The listing builds one solid part. Answer for the finished solid, in the listing's coordinates (mm). Face numbers are marked on the shaded views. A direction names the side the tool comes from. Coordinates: 2 decimals unless noted, no trailing zeros. Write each loop counter-clockwise with the first axis right and the second up, starting at its lowest first coordinate (ties: lowest second). Pieces come first, ordered by that corner, then holes.
(1) For a pull along Z with two mould halves and no side action, classify the marked faces 1, 2 and 3 as +Z half, -Z half, draft (parallel to the pull), parting line (faces both ways), or undercut.
(2) Which of the six approach directions +Z, -Z, +X, -X, +Y, -Y give full straight-line access (tool end or side, diameter ignored) to the marked faces 4 and 5?
(3) The part is cut by section A-A on x = -0.5. Determine the outline of the cut face in (y, z), plus the area to 3 significant figures.
(4) Straight lines are drawn through the part: line 1 (Z direction, x = -1, y = 0); line 2 (X direction, y = -5, z = 10.75). For each, find the intervals that lie inside material, in ascending order.
(5) Given P1, Ø9.5, axis at y = 2.5, z = 0.5, coming from the +X side; P2, Ø6, axis at x = 9, z = 0, coming from the -Y side; P3, Ø12, axis at x = 6, z = -10.5, coming from the -Y side; P4, Ø6, axis at x = 3, z = 9, coming from the -Y side, each flat-ended and moving along its own axis, determine where each tip first touches the part or whether it passes through.
from build123d import *

# Parameters (mm, degrees)
SKETCH_2_R      = 6.3
EXTRUDE_1_DEPTH = 1


with BuildPart() as part:
    # Эскиз1 → Повернуть-Тонкостенный3 (revolve)
    with BuildSketch(Plane.XY):
        Polygon((-41.34237999, 7), (16.65762001, 7), (19.313431248, 2.4), (27.313431248, 2.120633844), (27.2890016, 1.421060265), (18.901221633, 1.713967996), (16.253474821, 6.3), (-41.34237999, 6.3), align=None)
    revolve(axis=Axis((-11.565290599, 0, 0), (1, 0, 0)))

    # Эскиз2 → Бобышка-Вытянуть1 (add)
    with BuildSketch(Plane.ZY.offset(41.34237999)):
        with BuildLine():
            add(Edge.make_bspline(
                [(-14.5, 0), (-14.474728727, -1.250629482), (-14.242328004, -3.018058456), (-13.480726208, -5.156192857), (-12.386888331, -6.242148201), (-11.142838362, -6.727444369), (-9.562420274, -7.125179123), (-7.483693891, -7.691921698), (-4.724391308, -8.363720089), (-2.266989559, -9.122366404), (-0.655182959, -9.33281469), (-0.082845288, -9.355711433), (-2e-08, -9.357888542)],
                knots=[0, 0, 0, 0, 0.178779937, 0.255445115, 0.319697761, 0.392573489, 0.443879083, 0.553726464, 0.701162756, 0.851190942, 0.921407161, 0.933286403, 0.933286403, 0.933286403, 0.933286403], degree=3))
            add(Edge.make_bspline(
                [(14.5, 0), (14.474728734, -1.250629483), (14.242328006, -3.018058455), (13.480726218, -5.156192862), (12.386888336, -6.242148209), (11.142838364, -6.727444374), (9.562420275, -7.125179117), (7.483693885, -7.691921727), (4.724391348, -8.363719948), (2.266989446, -9.122366813), (0.655183079, -9.332814217), (0.082845248, -9.355711433), (-2e-08, -9.357888542)],
                knots=[0, 0, 0, 0, 0.178779937, 0.255445115, 0.319697761, 0.392573489, 0.443879083, 0.553726464, 0.701162756, 0.851190942, 0.921407161, 0.933286403, 0.933286403, 0.933286403, 0.933286403], degree=3))
            add(Edge.make_bspline(
                [(14.5, 0), (14.474728734, 1.250629483), (14.242328006, 3.018058455), (13.480726218, 5.156192862), (12.386888336, 6.242148209), (11.142838364, 6.727444374), (9.562420275, 7.125179117), (7.483693885, 7.691921727), (4.724391348, 8.363719948), (2.266989446, 9.122366813), (0.655183079, 9.332814217), (0.082845248, 9.355711433), (-2e-08, 9.357888542)],
                knots=[0, 0, 0, 0, 0.178779937, 0.255445115, 0.319697761, 0.392573489, 0.443879083, 0.553726464, 0.701162756, 0.851190942, 0.921407161, 0.933286403, 0.933286403, 0.933286403, 0.933286403], degree=3))
            add(Edge.make_bspline(
                [(-14.5, 0), (-14.474728727, 1.250629482), (-14.242328004, 3.018058456), (-13.480726208, 5.156192857), (-12.386888331, 6.242148201), (-11.142838362, 6.727444369), (-9.562420274, 7.125179123), (-7.483693891, 7.691921698), (-4.724391308, 8.363720089), (-2.266989559, 9.122366404), (-0.655182959, 9.33281469), (-0.082845288, 9.355711433), (-2e-08, 9.357888542)],
                knots=[0, 0, 0, 0, 0.178779937, 0.255445115, 0.319697761, 0.392573489, 0.443879083, 0.553726464, 0.701162756, 0.851190942, 0.921407161, 0.933286403, 0.933286403, 0.933286403, 0.933286403], degree=3))
        make_face()
        Circle(SKETCH_2_R, mode=Mode.SUBTRACT)
    extrude(amount=EXTRUDE_1_DEPTH)


solid = part.part
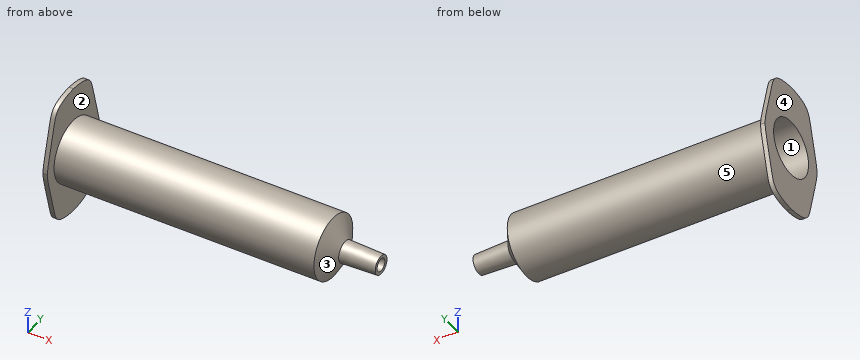
Model answer:
1. face 1: undercut
1. face 2: draft
1. face 3: parting line
2. face 4: +Z, -Z, -X, +Y, -Y
2. face 5: +X
3. outline: circle Ø14 at (0, 0); hole circle Ø12.6 at (0, 0)
3. area: 29.2 mm2
4. line 1: z = -7 to -6.3, 6.3 to 7
4. line 2: x = -42.34 to -41.34
5. P1: stops at x = 27.31
5. P2: stops at y = -7
5. P3: stops at y = -5.36
5. P4: stops at y = -3.61
